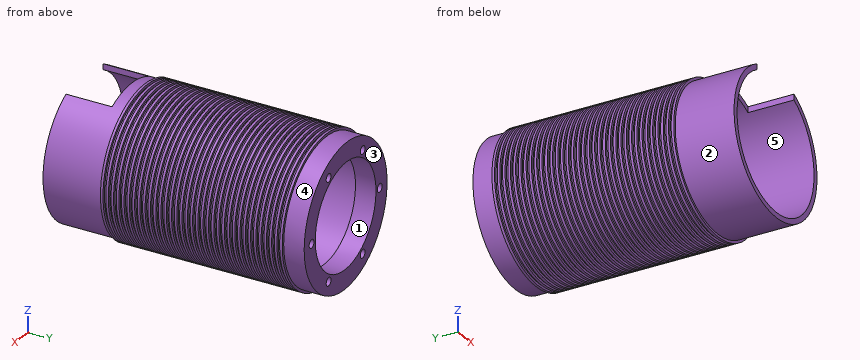
Solid Edge part; units mm, degrees
sketch "Sketch1" plane through (0, 0, 0) normal (0, -1, 0) x (1, 0, 0)
  circle A0 centre (0, 0) radius 28
  circle A1 centre (0, 0) radius 26
extrude "Protrusion1" add sketch "Sketch1" along normal mid plane 102
sketch "Sketch2" plane through (0, 0, 0) normal (1, 0, 0) x (0, 1, 0)
  line L0 (43, 28) -> (43, 29)
  line L1 (43, 29) -> (42, 29)
  line L2 (42, 29) -> (42, 28)
  line L3 (42, 28) -> (43, 28)
  dimension "D1" = 43
  dimension "D2" = 43
revolve "RevolvedProtrusion1" add sketch "Sketch2" angle 360 about axis through (0, 0, 0) along (0, 1, 0)
pattern_linear "Pattern1" count 35 spacing 2.0588 along (0, -1, 0) of "RevolvedProtrusion1"
sketch "Sketch3" plane through (0, 0, 0) normal (0, 0, 1) x (1, 0, 0)
  line L0 (-12.5, -51) -> (12.5, -51)
  line L1 (12.5, -51) -> (12.5, -33)
  line L2 (12.5, -33) -> (-12.5, -33)
  line L3 (-12.5, -33) -> (-12.5, -51)
  dimension "D1" = 12.5
  dimension "D2" = 12.5
extrude "Extrusionsausschnitt_1" cut sketch "Sketch3" along normal blind 55.2223
sketch "Sketch4" plane through (0, 51, 0) normal (0, 1, 0) x (0, 0, -1)
  circle A0 centre (0, 0) radius 20.5
  circle A1 centre (0, 0) radius 26
extrude "Extrusionsausprägung_2" add sketch "Sketch4" against normal blind 8
hole "Bohrung_1" at (11.5, 51, 19.9186) direction (0, -1, 0) diameter 3.242 depth 8
pattern_circular "Pattern2" count 6 over 360 about axis through (0, 51, 0) along (0, -1, 0) of "Bohrung_1"
properties material "Aluminiumlegierung:3.0205, Al 99.0, EN-AW 1200"
The model under review builds one solid part; all positions refer to its coordinate system, in mm. Face numbers are marked on the shaded views. A direction names the side the tool comes from. Give positions to 0.01 mm unless a question says otherwise; leave off trailing zeros. Answer in a Markdown table with one row per item. Add a question column.
1. Wall thickness on line 1 along Z through (x, y) = (1, 16.5); line 2 along X through (y, z) = (-3, 0.5); line 3 along X through (y, z) = (-12, -0.5): over which ranges is each line inside the solid? List them lowest first. Write a range as [from, to].
2. Draft analysis for pull direction X (two halves, no side actions). For the marked faces 3, 4 and 5, state which applies: +X half, -X half, draft (parallel to the pull), parting line (faces both ways), or undercut.
3. Insertion check: P1, Ø12, axis at x = -9, y = -21.5, coming from the -Z side; P2, Ø5, axis at y = -7.5, z = 5.5, coming from the -X side; P3, Ø5, axis at x = 6.5, y = 26.5, coming from the -Z side. Each pin has a flat end and moves straight along its axis. Give the tip position at first contact, or say it passes through.
4. Tool access review of the marked faces 1 and 2: name each direction out of +Z, -Z, +X, -X, +Y, -Y from which nothing blocks a thin tool from reaching the whole face with its end or side.
Ans:
| question | item | result |
|---|---|---|
| 1 | line 1 | z = [-27.98, -25.98], [25.98, 27.98] |
| 1 | line 2 | x = [-29, -26], [26, 29] |
| 1 | line 3 | x = [-28, -26], [26, 28] |
| 2 | face 3 | draft |
| 2 | face 4 | parting line |
| 2 | face 5 | undercut |
| 3 | P1 | stops at z = -28.84 |
| 3 | P2 | stops at x = -28.84 |
| 3 | P3 | stops at z = -28.72 |
| 4 | face 1 | +Y, -Y |
| 4 | face 2 | -Y |
